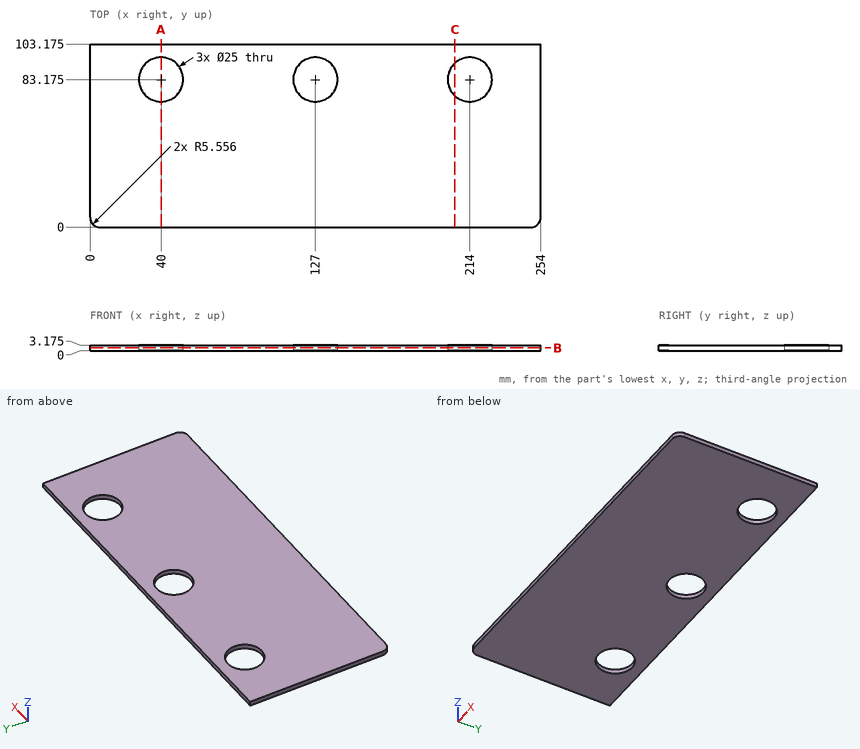
Here's the drawing with two shaded views (mm, measured from the low corner). I have some questions. Round coordinates to 2 decimals unless told otherwise and drop trailing zeros. Write each loop counter-clockwise with the first axis right and the second up, starting at its lowest first coordinate (ties: lowest second). Pieces come first, ordered by that corner, then holes.
(1) Suppose I cut it at B-B on z = 1.65. Write out the boundary of the cut face in (x, y) (1 decimal), and give its area (3 significant figures).
Findings below:
outline: (0, 5.6) arc R5.6 ccw to (5.6, 0) - (248.4, 0) arc R5.6 ccw to (254, 5.6) - (254, 103.2) - (0, 103.2) - close; hole circle Ø25 at (40, 83.2); hole circle Ø25 at (127, 83.2); hole circle Ø25 at (214, 83.2)
area: 24,700 mm2
(2) If I drill on probe 1 along Y at (x, z) = (40, 2.05) (1 decimal); probe 2 along X at (y, z) = (77, 1); probe 3 along Y at (x, z) = (31.5, 0.25) (1 decimal), over which ranges is the centre line in solid material (lowest first)?
Findings below:
probe 1: y = 0 to 70.7, 95.7 to 103.2
probe 2: x = 0 to 29.13, 50.87 to 116.13, 137.87 to 203.13, 224.87 to 254
probe 3: y = 0 to 74, 92.3 to 103.2
(3) Suppose I cut it at C-C on x = 205.5. Write out the boundary of the cut face in (y, z) (1 decimal).
Findings below:
outline: (0, 0) - (74, 0) - (74, 3.2) - (0, 3.2) - close; (92.3, 0) - (103.2, 0) - (103.2, 3.2) - (92.3, 3.2) - close
(4) Suppose I cut it at A-A on x = 40. Write out the boundary of the cut face in (y, z) (1 decimal).
Findings below:
outline: (0, 0) - (70.7, 0) - (70.7, 3.2) - (0, 3.2) - close; (95.7, 0) - (103.2, 0) - (103.2, 3.2) - (95.7, 3.2) - close
(5) For pin 1 (20 mm diameter, centred on x = 40, y = 83.175, fed in from +Z), with a flat end and sliding along its axis, tell me the tip position at first contact or that it passes through.
Findings below:
pin 1: passes through
